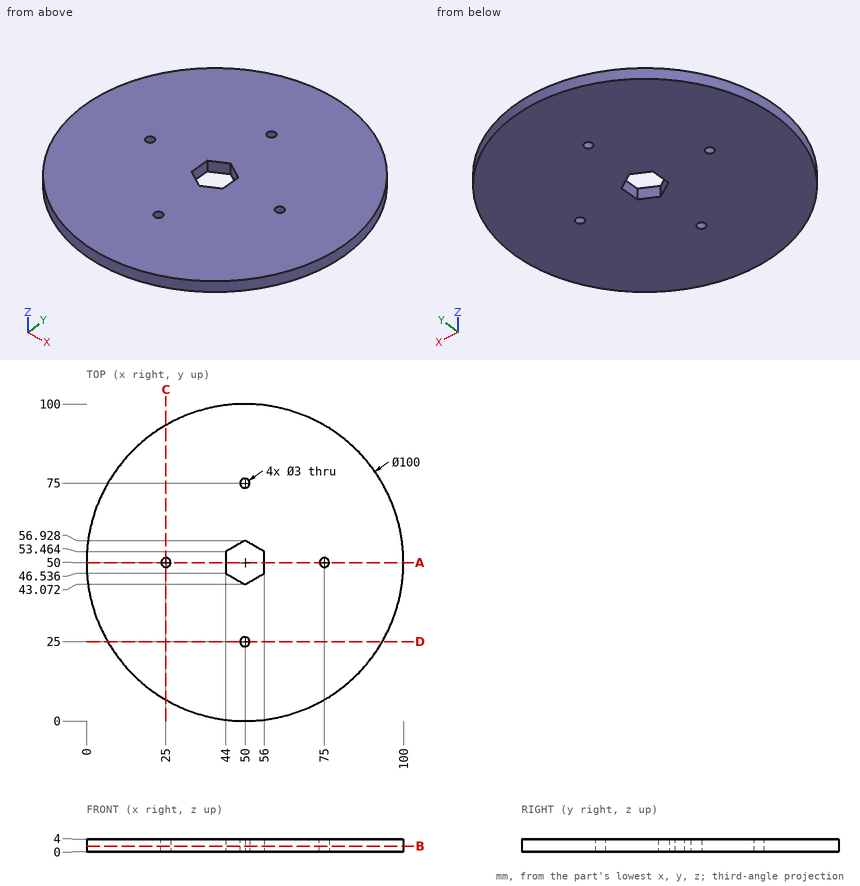
For this review, use the dimensioned drawing (mm, ordinates from the lowest corner) and the shaded views. Give positions to 0.01 mm unless a question says otherwise; leave off trailing zeros. Write each loop counter-clockwise with the first axis right and the second up, starting at its lowest first coordinate (ties: lowest second). Pieces come first, ordered by that corner, then holes. Notation, with made-up numbers: M 5.5,-6.5 L 59.5,-6.5 A14 cw 59.5,3.5 Z; hole C 71,82.5 d11. An arc over 180 degrees is marked long. Write item = value, one per line. Start each with the question number.
Q1. We need section A-A (y = 50). State the section outline as (x, z) points, plus the area to 3 significant figures.
Q2. Clearance check with flat-ended pins moving along their axes: pin 1 (2.5 mm diameter, centred on x = 50, y = 25, fed in from -Z); pin 2 (1.5 mm diameter, centred on y = 14.5, z = 2, fed in from -X). State where each tip first meets the part, or that it passes through.
Q3. We need section B-B (z = 1.75). State the section outline as (x, y) points, plus the area to 3 significant figures.
Q4. We need section C-C (x = 25). State the section outline as (y, z) points.
Q5. For line 1 (Y direction, x = 50, z = 2); line 2 (X direction, y = 75, z = 3); line 3 (Y direction, x = 46, z = 3.85), list the stretches that pass through material, from the lowest coordinate up.
Result set:
q1.outline = M 0,0 L 23.5,0 L 23.5,4 L 0,4 Z; M 26.5,0 L 44,0 L 44,4 L 26.5,4 Z; M 56,0 L 73.5,0 L 73.5,4 L 56,4 Z; M 76.5,0 L 100,0 L 100,4 L 76.5,4 Z
q1.area = 328 mm2
q2.pin_1 = through
q2.pin_2 = 14.05
q3.outline = C 50,50 d100; hole C 25,50 d3; hole M 44,46.54 L 50,43.07 L 56,46.54 L 56,53.46 L 50,56.93 L 44,53.46 Z; hole C 50,25 d3; hole C 50,75 d3; hole C 75,50 d3
q3.area = 7,700 mm2
q4.outline = M 6.7,0 L 48.5,0 L 48.5,4 L 6.7,4 Z; M 51.5,0 L 93.3,0 L 93.3,4 L 51.5,4 Z
q5.line_1 = 0 to 23.5, 26.5 to 43.07, 56.93 to 73.5, 76.5 to 100
q5.line_2 = 6.7 to 48.5, 51.5 to 93.3
q5.line_3 = 0.16 to 45.38, 54.62 to 99.84
